Design review of the part built by this model. Coordinates are the model's own, in mm. A direction names the side the tool comes from. Coordinates: 2 decimals unless noted, no trailing zeros. Write each loop counter-clockwise with the first axis right and the second up, starting at its lowest first coordinate (ties: lowest second). Pieces come first, ordered by that corner, then holes. Notation, with made-up numbers: (54, -14) -> (64, -14) arc R33 ccw to (64, 18) -> close; hole circle Ø4 at (80.25, 9). An arc over 180 degrees is marked (long way). Answer in a Markdown table with one row per item. Add a question column.
Item 1: To check wall thickness, follow line 1 (Y direction, x = 58.75, z = 22.86); line 2 (Z direction, x = 12, y = 68.5); line 3 (Y direction, x = 50.5, z = 32). State the ranges of each line that lie inside material, in increasing order.
Item 2: Take a section at D-D, the plane x = 16.5. Write out the cut boundary in (y, z), and give its area (3 significant figures).
Item 3: Take a section at A-A, the plane x = -53. Write out the cut boundary in (y, z), and give its area (3 significant figures).
Item 4: Draft analysis for pull direction Z (two halves, no side actions). For faces 1 (the face through (-63.5, 5, 17)), 2 (the face through (7, -30, 0)), 3 (the face through (-55.987, 0.279, 16.516)), state which applies: released by +Z, released by -Z, zero draft, split by the parting line, or undercut.
Item 5: For faces 4 (the face through (-1, 22.86, 23)), 5 (the face through (-1, -22.86, 23)), 6 (the face through (44, 0, 0)), 7 (the face through (-38, 0, 0)), 8 (the face through (55.987, 0.279, 29.204)), list the 3-axis set-ups (+Z, -Z, +X, -X, +Y, -Y) from which the entire face can be reached by the end or side of a thin tool; tool diameter is ignored.
Item 6: Take a section at B-B, the plane z = 22.86. Write out the cut boundary in (x, y).
Item 7: Take a section at C-C, the plane y = 0. Write out the cut boundary in (x, z).
Item 8: Clearance check with flat-ended pins moving along their axes: P1, Ø10, axis at y = -15, z = -6, coming from the +X side; P2, Ø23, axis at x = -15.5, z = 19.5, coming from the -Y side; P3, Ø10, axis at y = 0, z = 22.86, coming from the +X side. State where each tip first meets the part, or that it passes through.
from build123d import *

# Parameters (mm, degrees)
SKETCH1_W           = 127
SKETCH1_H           = 45.72
BOSS_EXTRUDE1_DEPTH = 45.72
SKETCH2_W           = 38.1
SKETCH2_H           = 228.6
BOSS_EXTRUDE2_DEPTH = 56.388
SKETCH3_R           = 6.35
CUT_EXTRUDE1_DEPTH  = 15.24
SKETCH4_R           = 6.35
CUT_EXTRUDE2_DEPTH  = 15.24


with BuildPart() as part:
    # Sketch1 → Boss-Extrude1 (new body)
    with BuildSketch(Plane.XY):
        Rectangle(SKETCH1_W, SKETCH1_H)
    extrude(amount=BOSS_EXTRUDE1_DEPTH)

    # Sketch2 → Boss-Extrude2 (add)
    with BuildSketch(Plane(origin=(0, 0, 0), x_dir=(-1, 0, 0), z_dir=(0, 0, -1))):
        with Locations((-6.276150489, 76.2)):
            Rectangle(SKETCH2_W, SKETCH2_H)
    extrude(amount=BOSS_EXTRUDE2_DEPTH)

    # Sketch3 → Cut-Extrude1 (cut)
    with BuildSketch(Plane(origin=(63.5, 0, 0), x_dir=(0, 0, -1), z_dir=(1, 0, 0))):
        with Locations((-22.86, 0)):
            Circle(SKETCH3_R)
    extrude(amount=-CUT_EXTRUDE1_DEPTH, mode=Mode.SUBTRACT)

    # Sketch4 → Cut-Extrude2 (cut)
    with BuildSketch(Plane.ZY.offset(63.5)):
        with Locations((22.86, 0)):
            Circle(SKETCH4_R)
    extrude(amount=-CUT_EXTRUDE2_DEPTH, mode=Mode.SUBTRACT)


solid = part.part
Answers:
| question | item | result |
|---|---|---|
| 1 | line 1 | y = -22.86 to -6.35, 6.35 to 22.86 |
| 1 | line 2 | z = -56.39 to 0 |
| 1 | line 3 | y = -22.86 to 22.86 |
| 2 | outline | (-38.1, -56.39) -> (190.5, -56.39) -> (190.5, 0) -> (22.86, 0) -> (22.86, 45.72) -> (-22.86, 45.72) -> (-22.86, 0) -> (-38.1, 0) -> close |
| 2 | area | 15,000 mm^2 |
| 3 | outline | (-22.86, 0) -> (22.86, 0) -> (22.86, 45.72) -> (-22.86, 45.72) -> close; hole circle Ø12.7 at (0, 22.86) |
| 3 | area | 1,960 mm^2 |
| 4 | face 1 | zero draft |
| 4 | face 2 | released by +Z |
| 4 | face 3 | undercut |
| 5 | face 4 | +Z, +X, -X, +Y |
| 5 | face 5 | +Z, +X, -X, -Y |
| 5 | face 6 | -Z, +X, +Y, -Y |
| 5 | face 7 | -Z, -X, +Y, -Y |
| 5 | face 8 | +X |
| 6 | outline | (-63.5, -22.86) -> (63.5, -22.86) -> (63.5, -6.35) -> (48.26, -6.35) -> (48.26, 6.35) -> (63.5, 6.35) -> (63.5, 22.86) -> (-63.5, 22.86) -> (-63.5, 6.35) -> (-48.26, 6.35) -> (-48.26, -6.35) -> (-63.5, -6.35) -> close |
| 7 | outline | (-63.5, 0) -> (-12.77, 0) -> (-12.77, -56.39) -> (25.33, -56.39) -> (25.33, 0) -> (63.5, 0) -> (63.5, 16.51) -> (48.26, 16.51) -> (48.26, 29.21) -> (63.5, 29.21) -> (63.5, 45.72) -> (-63.5, 45.72) -> (-63.5, 29.21) -> (-48.26, 29.21) -> (-48.26, 16.51) -> (-63.5, 16.51) -> close |
| 8 | P1 | stops at x = 25.33 |
| 8 | P2 | stops at y = -22.86 |
| 8 | P3 | stops at x = 48.26 |
